```python
from build123d import *

# Parameters (mm, degrees)
SKETCH_1_R               = 39.75
EXTRUDE_1_DEPTH          = 10
SKETCH_2_R               = 18.25
CUT_EXTRUDE_1_DEPTH      = 4
SKETCH_3_R               = 11.5
CUT_EXTRUDE_2_DEPTH      = 2
SKETCH_4_R               = 1.5
CUT_EXTRUDE_3_DEPTH      = 6
SKETCH_5_R               = 3
CUT_EXTRUDE_4_DEPTH      = 2
SKETCH_7_R               = 2.65
CUT_EXTRUDE_5_DEPTH      = 8
PATTERN_CIRCULAR_1_COUNT = 2
PATTERN_CIRCULAR_1_ANGLE = 25
F_1_THE_OTHER_WAY_COUNT  = 2
F_1_THE_OTHER_WAY_ANGLE  = 25
MIRROR_1_COPY_1_SKETCH_R = 2.65
MIRROR_1_COPY_1_DEPTH    = 8
MIRROR_1_COPY_2_SKETCH_R = 2.65
MIRROR_1_COPY_2_DEPTH    = 8
SKETCH_8_R               = 10
CUT_EXTRUDE_6_DEPTH      = 4
SKETCH_9_R               = 2.65
CUT_EXTRUDE_7_DEPTH      = 8
PATTERN_CIRCULAR_2_COUNT = 2
EXTRUDE_START            = 5
SKETCH_10_R              = 23.25
SKETCH_10_R_2            = 18.25
EXTRUDE_2_DEPTH          = 5
CUT_EXTRUDE_START        = -10
CUT_EXTRUDE_8_DEPTH      = 10
FILLET_1_R               = 1


# Read off the part's stored shape, not the designer's step: Вырез-Вытянуть8
with BuildPart() as part:
    # Эскиз1 → Бобышка-Вытянуть1 (new body)
    with BuildSketch(Plane.XY):
        Circle(SKETCH_1_R)
    extrude(amount=EXTRUDE_1_DEPTH)

    # Эскиз2 → Вырез-Вытянуть1 (cut)
    with BuildSketch(Plane.XY.offset(10)):
        Circle(SKETCH_2_R)
    extrude(amount=-CUT_EXTRUDE_1_DEPTH, mode=Mode.SUBTRACT)

    # Эскиз3 → Вырез-Вытянуть2 (cut)
    with BuildSketch(Plane.XY.offset(6)):
        Circle(SKETCH_3_R)
    extrude(amount=-CUT_EXTRUDE_2_DEPTH, mode=Mode.SUBTRACT)

    # Эскиз4 → Вырез-Вытянуть3 (cut)
    with BuildSketch(Plane.XY.offset(6)):
        with Locations((-9.899494937, 9.899494937)):
            Circle(SKETCH_4_R)
        with Locations((9.899494937, 9.899494937)):
            Circle(SKETCH_4_R)
        with Locations((9.899494937, -9.899494937)):
            Circle(SKETCH_4_R)
        with Locations((-9.899494937, -9.899494937)):
            Circle(SKETCH_4_R)
    extrude(amount=-CUT_EXTRUDE_3_DEPTH, mode=Mode.SUBTRACT)

    # Эскиз5 → Вырез-Вытянуть4 (cut)
    with BuildSketch(Plane(origin=(0, 0, 0), x_dir=(-1, 0, 0), z_dir=(0, 0, -1))):
        with Locations((-9.899494937, 9.899494937)):
            Circle(SKETCH_5_R)
        with Locations((9.899494937, 9.899494937)):
            Circle(SKETCH_5_R)
        with Locations((9.899494937, -9.899494937)):
            Circle(SKETCH_5_R)
        with Locations((-9.899494937, -9.899494937)):
            Circle(SKETCH_5_R)
    extrude(amount=-CUT_EXTRUDE_4_DEPTH, mode=Mode.SUBTRACT)

    # Эскиз7 → Вырез-Вытянуть5 (cut)
    with BuildSketch(Plane(origin=(0, 39.75, 0), x_dir=(0, 0, -1), z_dir=(0, 1, 0))):
        with Locations(Location((-5, 0, 0), (0, 0, 90))):
            Circle(SKETCH_7_R)
    cut_extrude_5 = extrude(amount=-CUT_EXTRUDE_5_DEPTH, mode=Mode.SUBTRACT)

    # Круговой массив1: Вырез-Вытянуть5 ×2 about axis
    pattern_circular_1_axis = Axis((0, 0, 10), (0, 0, -1))
    for i in range(1, PATTERN_CIRCULAR_1_COUNT):
        add(cut_extrude_5.rotate(pattern_circular_1_axis, i * PATTERN_CIRCULAR_1_ANGLE / (PATTERN_CIRCULAR_1_COUNT - 1)), mode=Mode.SUBTRACT)

    # 1 the other way: Вырез-Вытянуть5 ×2 about axis
    f_1_the_other_way_axis = Axis((0, 0, 10), (0, 0, 1))
    for i in range(1, F_1_THE_OTHER_WAY_COUNT):
        add(cut_extrude_5.rotate(f_1_the_other_way_axis, i * F_1_THE_OTHER_WAY_ANGLE / (F_1_THE_OTHER_WAY_COUNT - 1)), mode=Mode.SUBTRACT)

    # Зеркальное отражение1: Вырез-Вытянуть5 across plane
    add(cut_extrude_5.mirror(Plane.ZX), mode=Mode.SUBTRACT)

    # Зеркальное отражение1 copy 1 sketch → Зеркальное отражение1 copy 1 (cut)
    with BuildSketch(Plane(origin=(16.799075904, -36.025734535, 0), x_dir=(0, 0, -1), z_dir=(0.4226182617407035, -0.906307787036648, 0))):
        with Locations((-5, 0)):
            Circle(MIRROR_1_COPY_1_SKETCH_R)
    extrude(amount=-MIRROR_1_COPY_1_DEPTH, mode=Mode.SUBTRACT)

    # Зеркальное отражение1 copy 2 sketch → Зеркальное отражение1 copy 2 (cut)
    with BuildSketch(Plane(origin=(-16.799075904, -36.025734535, 0), x_dir=(0, 0, -1), z_dir=(-0.42261826174069717, -0.9063077870366509, 0))):
        with Locations((-5, 0)):
            Circle(MIRROR_1_COPY_2_SKETCH_R)
    extrude(amount=-MIRROR_1_COPY_2_DEPTH, mode=Mode.SUBTRACT)

    # Эскиз8 → Вырез-Вытянуть6 (cut)
    with BuildSketch(Plane.XY.offset(4)):
        Circle(SKETCH_8_R)
    extrude(amount=-CUT_EXTRUDE_6_DEPTH, mode=Mode.SUBTRACT)

    # Эскиз9 → Вырез-Вытянуть7 (cut)
    with BuildSketch(Plane.ZY.offset(39.75)):
        with Locations((5, 0)):
            Circle(SKETCH_9_R)
    cut_extrude_7 = extrude(amount=-CUT_EXTRUDE_7_DEPTH, mode=Mode.SUBTRACT)

    # Круговой массив2: Вырез-Вытянуть7 ×2 about axis
    pattern_circular_2_axis = Axis((0, 0, 10), (0, 0, -1))
    for i in range(1, PATTERN_CIRCULAR_2_COUNT):
        add(cut_extrude_7.rotate(pattern_circular_2_axis, i * 360 / PATTERN_CIRCULAR_2_COUNT), mode=Mode.SUBTRACT)

    # Эскиз10 → Бобышка-Вытянуть2 (add)
    with BuildSketch(Plane.XY.offset(10).offset(EXTRUDE_START)):
        Circle(SKETCH_10_R)
        Circle(SKETCH_10_R_2, mode=Mode.SUBTRACT)
    extrude(amount=-EXTRUDE_2_DEPTH)

    # Вырез-Вытянуть8 outline → Вырез-Вытянуть8 (cut)
    with BuildSketch(Plane(origin=(0, 0, 0), x_dir=(-1, 0, 0), z_dir=(0, 0, -1)).offset(CUT_EXTRUDE_START)):
        with BuildLine():
            Line((36.811173575, 15), (26.811173575, 15))
            Line((26.811173575, 15), (26.811173575, -15))
            Line((26.811173575, -15), (36.811173575, -15))
            ThreePointArc((36.811173575, -15), (39.75, 0), (36.811173575, 15))
        make_face()
    extrude(amount=CUT_EXTRUDE_8_DEPTH, mode=Mode.SUBTRACT)

    # Скругление1
    fillet_1_edges = [part.edges().sort_by_distance(p)[0] for p in [
        (-26.811173575, 15, 5),
        (-26.811173575, -15, 5),
        (-36.811173575, -15, 5),
        (-36.811173575, 15, 5),
    ]]
    fillet(fillet_1_edges, radius=FILLET_1_R)


solid = part.part
```
Verification items for the finished model (mm, model axes). A direction names the side the tool comes from. Round coordinates to 2 decimals unless told otherwise and drop trailing zeros. Write each loop counter-clockwise with the first axis right and the second up, starting at its lowest first coordinate (ties: lowest second). Pieces come first, ordered by that corner, then holes. Notation, with made-up numbers: (-19.5, 43.25) - (-0.5, 43.25) arc R29 ccw to (-0.5, 69.25) - close; hole circle Ø7 at (48.5, 54.25). An arc over 180 degrees is marked (long way). Answer as a JSON object with one key per item and string values. Group by question number.
Q1. Thickness scan on line 1 (Y direction, x = -14, z = 4.5); line 2 (X direction, y = -11, z = 3); line 3 (Z direction, x = 20, y = 12.5). Record the ranges inside material, lowest first.
Q2. Section check C-C, the plane z = 11.5. Enter the section's corners in (x, y), plus the area to 3 significant figures.
Q3. Mould release check, pull along Y, two halves, no side actions. Record for faces 4 (the flat face through (18, -17, 10)), 5 (the flat face through (0, -31.75, 5)), 6 (the flat face through (0, 31.75, 5)), 7 (the flat face through (13.45, 28.76, 5.04)): released by +Y, released by -Y, zero draft, split by the parting line, or undercut.
Q4. Section check A-A, the plane x = 0. Enter the section's corners in (y, z).
Q5. Section check B-B, the plane y = -19.5. Enter the section's corners in (x, z), plus the area to 3 significant figures.
Q6. Tool access check on faces 1 (the flat face through (-26.811, 0, 5)), 2 (the flat face through (13.45, -28.76, 5.04)), 3 (the cylindrical face through (35.806, -0.796, 7.528)). Record the directions out of +Z, -Z, +X, -X, +Y, -Y that give a thin tool (end or side, any length) a straight path to the whole face; none if there is none.
Q7. Section check D-D, the plane z = 5. Give the number of separate pieces and of enclosed holes in the cut face, plus the area to 3 significant figures.
Q8. Go/stop test with flat-tipped pins: pin 1 Ø20.5 at (x, y) = (0, 0) entering from -Z; pin 2 Ø2 at (x, z) = (-15, 5) entering from +Y; pin 3 Ø3.5 at (x, y) = (9.9, 9.9) entering from +Z; pin 4 Ø1.5 at (x, z) = (13.5, 6) entering from -Y. Record where each tip stops, or that it passes through.
Found:
{
 "1": {"line 1": "y = -37.2 to -36.18, -28.5 to 28.5, 36.18 to 37.2", "line 2": "x = -26.81 to -10.92, -8.88 to 8.88, 10.92 to 38.2", "line 3": "z = 0 to 10"},
 "2": {"outline": "circle Ø46.5 at (0, 0); hole circle Ø36.5 at (0, 0)", "area": "652 mm^2"},
 "3": {"face 4": "zero draft", "face 5": "released by -Y", "face 6": "released by +Y", "face 7": "undercut"},
 "4": {"outline": "(-39.75, 0) - (-10, 0) - (-10, 4) - (-11.5, 4) - (-11.5, 6) - (-18.25, 6) - (-18.25, 15) - (-23.25, 15) - (-23.25, 10) - (-39.75, 10) - (-39.75, 7.65) - (-31.75, 7.65) - (-31.75, 2.35) - (-39.75, 2.35) - close; (10, 0) - (39.75, 0) - (39.75, 2.35) - (31.75, 2.35) - (31.75, 7.65) - (39.75, 7.65) - (39.75, 10) - (23.25, 10) - (23.25, 15) - (18.25, 15) - (18.25, 6) - (11.5, 6) - (11.5, 4) - (10, 4) - close"},
 "5": {"outline": "(-34.64, 0) - (34.64, 0) - (34.64, 10) - (12.66, 10) - (12.66, 15) - (-12.66, 15) - (-12.66, 10) - (-34.64, 10) - close", "area": "819 mm^2"},
 "6": {"face 1": "+Z, -Z, -X", "face 2": "none", "face 3": "+X"},
 "7": {"separate pieces": "1", "enclosed holes": "5", "area": "3,860 mm^2"},
 "8": {"pin 1": "stops at z = 0", "pin 2": "stops at y = 37.2", "pin 3": "stops at z = 6", "pin 4": "stops at y = -37.65"}
}
